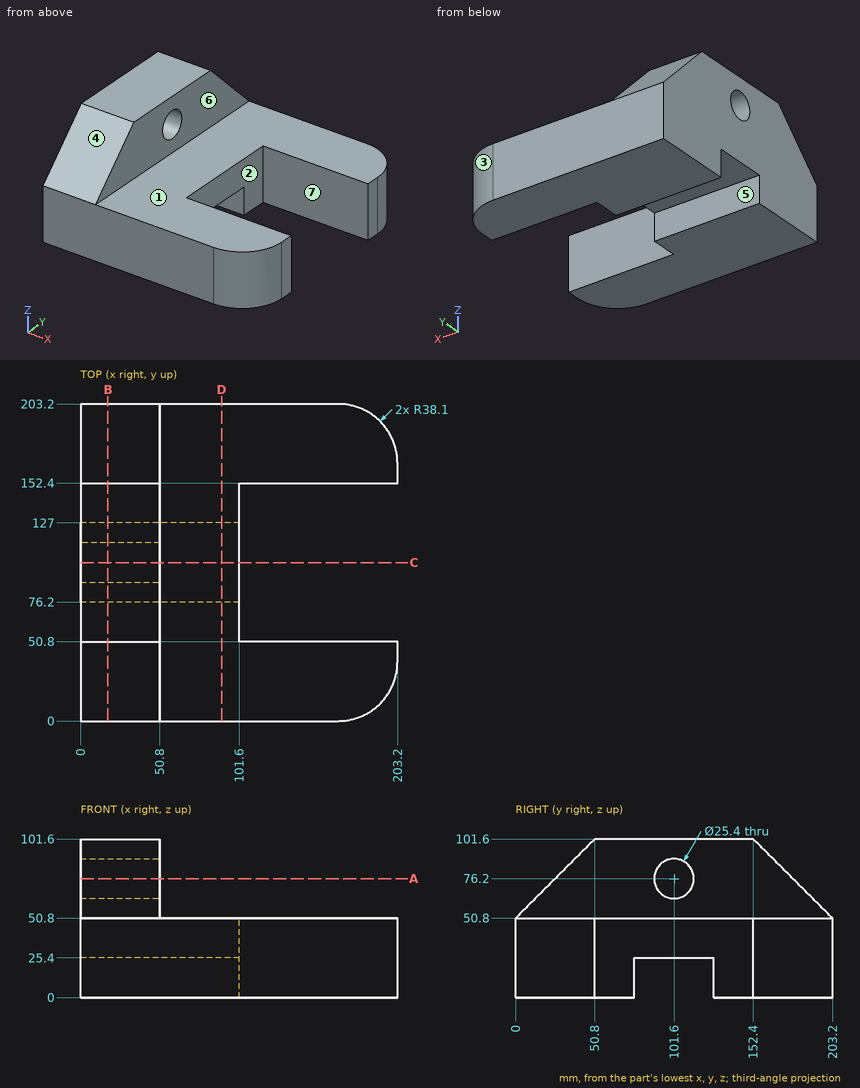
Could you check a few things on this drawing? It's one solid part, dimensions in mm from its lowest x, y, z. A direction names the side the tool comes from. Give positions to 0.01 mm unless a question says otherwise; leave off trailing zeros. Order: outer loops, then holes, each group sorted by start corner. A loop starts at its lowest first (then second) coordinate and runs counter-clockwise, first axis right, second up. Notation, with made-up numbers: (32.5, -27.5) - (48.5, -27.5) arc R14 ccw to (48.5, -14.5) - close; hole circle Ø6 at (86, 77.5). An arc over 180 degrees is marked (long way). One line per item, written item: value. Start each with the question number.
1. Imagine slicing it at D-D on x = 90.5. List the corners of the cut face in (y, z) for me.
2. For P1, Ø15, axis at y = 121.5, z = 33.5, coming from the +X side; P2, Ø4, axis at x = 178, y = 30, coming from the +Z side; P3, Ø15, axis at x = 56.5, y = 105, coming from the -Z side, each with a flat end and sliding along its axis, tell me the tip position at first contact or that it passes through.
3. Thinking about a two-plate mould opening in Y: for the marked faces 1, 2 and 3, which applies, +Y half, -Y half, draft (parallel to the pull), parting line (faces both ways), or undercut?
4. Imagine slicing it at A-A on z = 76.2. List the corners of the cut face in (x, y) for me.
5. If I drill on probe 1 along Z at (x, y) = (22, 101); probe 2 along Z at (x, y) = (94, 34.5); probe 3 along X at (y, z) = (140.5, 24.5), over which ranges is the centre line in solid material (lowest first)?
6. Imagine slicing it at B-B on x = 17.5. List the corners of the cut face in (y, z) for me, plus the area to 3 significant figures.
7. For the marked faces 4, 5, 6 and 7, which set-ups out of +Z, -Z, +X, -X, +Y, -Y let a thin tool reach every point of the face, with its end or its side?
8. Imagine slicing it at C-C on y = 101.6. List the corners of the cut face in (x, z) for me.
Values:
1. outline: (0, 0) - (76.2, 0) - (76.2, 25.4) - (127, 25.4) - (127, 0) - (203.2, 0) - (203.2, 50.8) - (0, 50.8) - close
2. P1: x = 101.6
2. P2: z = 50.8
2. P3: z = 25.4
3. face 1: draft
3. face 2: undercut
3. face 3: +Y half
4. outline: (0, 25.4) - (50.8, 25.4) - (50.8, 88.9) - (0, 88.9) - close; (0, 114.3) - (50.8, 114.3) - (50.8, 177.8) - (0, 177.8) - close
5. probe 1: 25.4 to 63.51, 88.89 to 101.6
5. probe 2: 0 to 50.8
5. probe 3: 0 to 101.6
6. outline: (0, 0) - (76.2, 0) - (76.2, 25.4) - (127, 25.4) - (127, 0) - (203.2, 0) - (203.2, 50.8) - (152.4, 101.6) - (50.8, 101.6) - (0, 50.8) - close; hole circle Ø25.4 at (101.6, 76.2)
6. area: 16,300 mm²
7. face 4: +Z, +X, -X, -Y
7. face 5: -Z, +X, -X
7. face 6: +Z, +X, +Y, -Y
7. face 7: +Z, -Z, +X
8. outline: (0, 25.4) - (101.6, 25.4) - (101.6, 50.8) - (50.8, 50.8) - (50.8, 63.5) - (0, 63.5) - close; (0, 88.9) - (50.8, 88.9) - (50.8, 101.6) - (0, 101.6) - close
